Drawing for the job (mm, zero at the part's lowest x, y, z). A direction names the side the tool comes from. Round coordinates to 2 decimals unless told otherwise and drop trailing zeros. Write each loop counter-clockwise with the first axis right and the second up, starting at its lowest first coordinate (ties: lowest second). Pieces come first, ordered by that corner, then holes. Notation, with made-up numbers: M 8,55 L 44,55 A28 cw 44,85 Z; hole C 54.25,87 d5. An arc over 180 degrees is marked long. Use a Markdown table: item, result. Add a question column.
1) Which spindle directions (+Z, -Z, +X, -X, +Y, -Y) get a long thin tool onto all of the face, cutting with end or side? Do the marked faces 1, 2 and 3. Say none if no direction does.
2) Slice it at D-D on x = 30.7. Write the cut outline in (y, z).
3) Drop a flat-ended pin along its axis: P1, Ø1.2, axis at x = 32, z = 2, coming from the -Y side. Give the stop position or say it passes through.
4) Slice it at A-A on x = 18. Write the cut outline in (y, z), plus the area to 3 significant figures.
5) Two-plate mould, pull along X, no slides. Class the marked faces 4, 5 and 6: released by +X, released by -X, zero draft, split by the parting line, or undercut.
6) Slice it at C-C on z = 1.95. Write the cut outline in (x, y).
7) Wall check: probe 1 along Y at (x, z) = (18, 1.4); probe 2 along Y at (x, z) = (17.5, 3.75); probe 3 along Y at (x, z) = (5.3, 2). Give the ranges that are in metal, low to high.
8) Slice it at B-B on y = 28. Write the cut outline in (x, z).
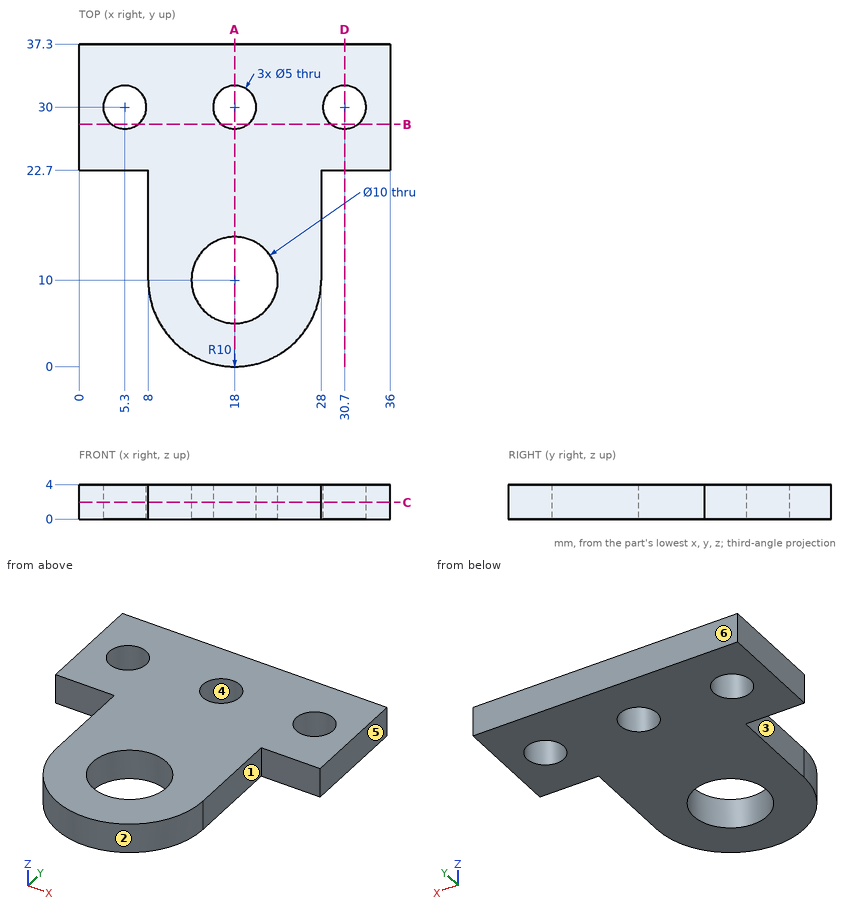
Entries:
| question | item | result |
|---|---|---|
| 1 | face 1 | +Z, -Z, +X, -Y |
| 1 | face 2 | +Z, -Z, -Y |
| 1 | face 3 | +Z, -Z, -X, -Y |
| 2 | outline | M 22.7,0 L 27.5,0 L 27.5,4 L 22.7,4 Z; M 32.5,0 L 37.3,0 L 37.3,4 L 32.5,4 Z |
| 3 | P1 | stops at y = 22.7 |
| 4 | outline | M 0,0 L 5,0 L 5,4 L 0,4 Z; M 15,0 L 27.5,0 L 27.5,4 L 15,4 Z; M 32.5,0 L 37.3,0 L 37.3,4 L 32.5,4 Z |
| 4 | area | 89.2 mm^2 |
| 5 | face 4 | undercut |
| 5 | face 5 | released by +X |
| 5 | face 6 | zero draft |
| 6 | outline | M 0,22.7 L 8,22.7 L 8,10 A10 ccw 28,10 L 28,22.7 L 36,22.7 L 36,37.3 L 0,37.3 Z; hole C 5.3,30 d5; hole C 18,10 d10; hole C 18,30 d5; hole C 30.7,30 d5 |
| 7 | probe 1 | y = 0 to 5, 15 to 27.5, 32.5 to 37.3 |
| 7 | probe 2 | y = 0.01 to 5.03, 14.97 to 27.55, 32.45 to 37.3 |
| 7 | probe 3 | y = 22.7 to 27.5, 32.5 to 37.3 |
| 8 | outline | M 0,0 L 3.8,0 L 3.8,4 L 0,4 Z; M 6.8,0 L 16.5,0 L 16.5,4 L 6.8,4 Z; M 19.5,0 L 29.2,0 L 29.2,4 L 19.5,4 Z; M 32.2,0 L 36,0 L 36,4 L 32.2,4 Z |
